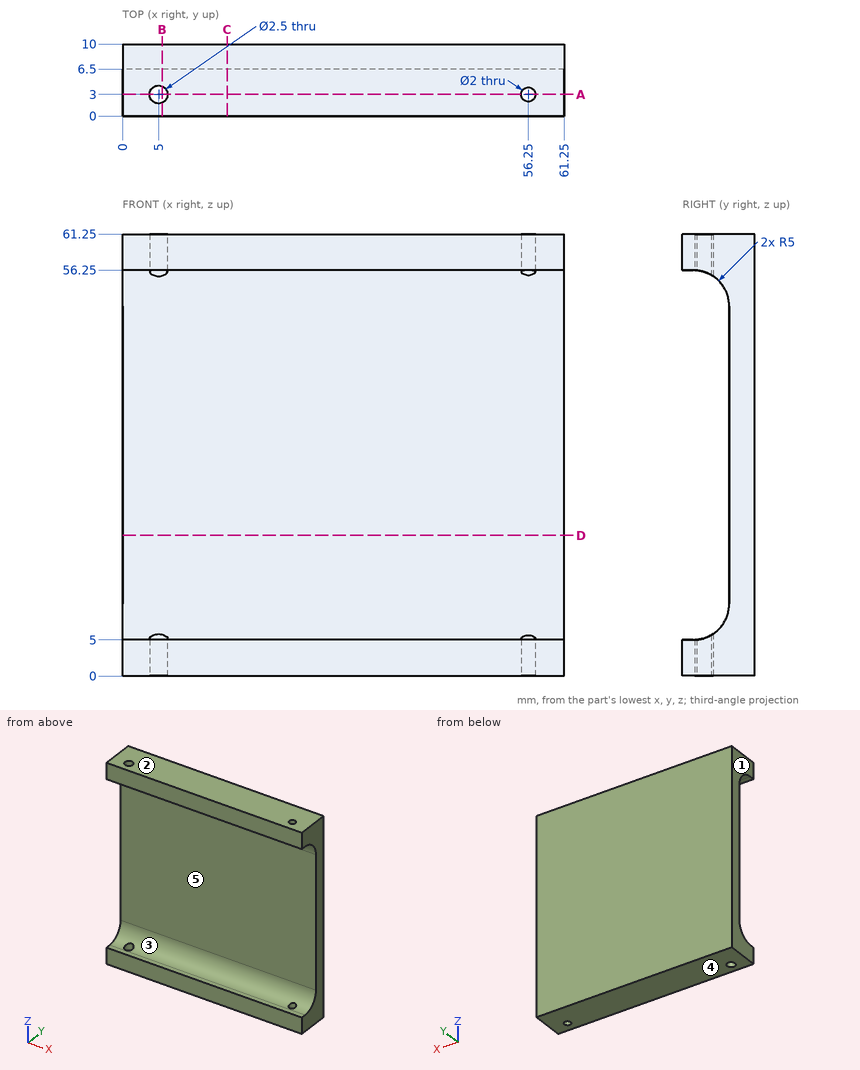
Design review of the part shown in the three views and the two pictorial views. Dimensions are in mm from the part's minimum x, y and z. A direction names the side the tool comes from. Round coordinates to 2 decimals unless told otherwise and drop trailing zeros. Order: outer loops, then holes, each group sorted by start corner. A loop starts at its lowest first (then second) coordinate and runs counter-clockwise, first axis right, second up.
(1) Take a section at C-C, the plane x = 14.5. State the section outline as (y, z) points.
Working result:
outline: (0, 0) - (10, 0) - (10, 61.25) - (0, 61.25) - (0, 56.25) - (1.5, 56.25) arc R5 cw to (6.5, 51.25) - (6.5, 10) arc R5 cw to (1.5, 5) - (0, 5) - close
(2) Mouldability with a two-part tool opening along Z and no side actions: class the marked faces 1, 2 and 3 as released by +Z, released by -Z, zero draft, split by the parting line, or undercut.
Working result:
face 1: zero draft
face 2: released by +Z
face 3: undercut
(3) Take a section at B-B, the plane x = 5.5. State the section outline as (y, z) points.
Working result:
outline: (0, 0) - (1.85, 0) - (1.85, 5.01) arc R5 cw to (1.5, 5) - (0, 5) - close; (0, 56.25) - (1.5, 56.25) arc R5 cw to (1.85, 56.24) - (1.85, 61.25) - (0, 61.25) - close; (4.15, 0) - (10, 0) - (10, 61.25) - (4.15, 61.25) - (4.15, 55.49) arc R5 cw to (6.5, 51.25) - (6.5, 10) arc R5 cw to (4.15, 5.76) - close
(4) Take a section at A-A, the plane y = 3. State the section outline as (x, z) points.
Working result:
outline: (0, 0) - (3.75, 0) - (3.75, 5.23) - (0, 5.23) - close; (0, 56.02) - (3.75, 56.02) - (3.75, 61.25) - (0, 61.25) - close; (6.25, 0) - (55.25, 0) - (55.25, 5.23) - (6.25, 5.23) - close; (6.25, 56.02) - (55.25, 56.02) - (55.25, 61.25) - (6.25, 61.25) - close; (57.25, 0) - (61.25, 0) - (61.25, 5.23) - (57.25, 5.23) - close; (57.25, 56.02) - (61.25, 56.02) - (61.25, 61.25) - (57.25, 61.25) - close
(5) Take a section at D-D, the plane z = 19.5. State the section outline as (x, y) points, plus the area to 3 significant figures.
Working result:
outline: (0, 6.5) - (61.25, 6.5) - (61.25, 10) - (0, 10) - close
area: 214 mm2
(6) Wall thickness on L1, parallel to X at y = 3, z = 59.25; L2, parallel to Z at x = 58, y = 1; L3, parallel to Y at x = 5, z = 59.85: over which ranges is each line inside the solid? List them lowest first.
Working result:
L1: x = 0 to 3.75, 6.25 to 55.25, 57.25 to 61.25
L2: z = 0 to 5, 56.25 to 61.25
L3: y = 0 to 1.75, 4.25 to 10
(7) Tool access review of the marked faces 4 and 5: name each direction out of +Z, -Z, +X, -X, +Y, -Y from which nothing blocks a thin tool from reaching the whole face with its end or side.
Working result:
face 4: -Z, +X, -X, +Y, -Y
face 5: +X, -X, -Y
(8) For P1, Ø4, axis at x = 50.5, z = 36.5, coming from the -Y side; P2, Ø1.5, axis at x = 50, z = 8.5, coming from the -Y side, all flat-tipped, find the tip position at first contact; note any pin that passes through.
Working result:
P1: stops at y = 6.5
P2: stops at y = 5.97
